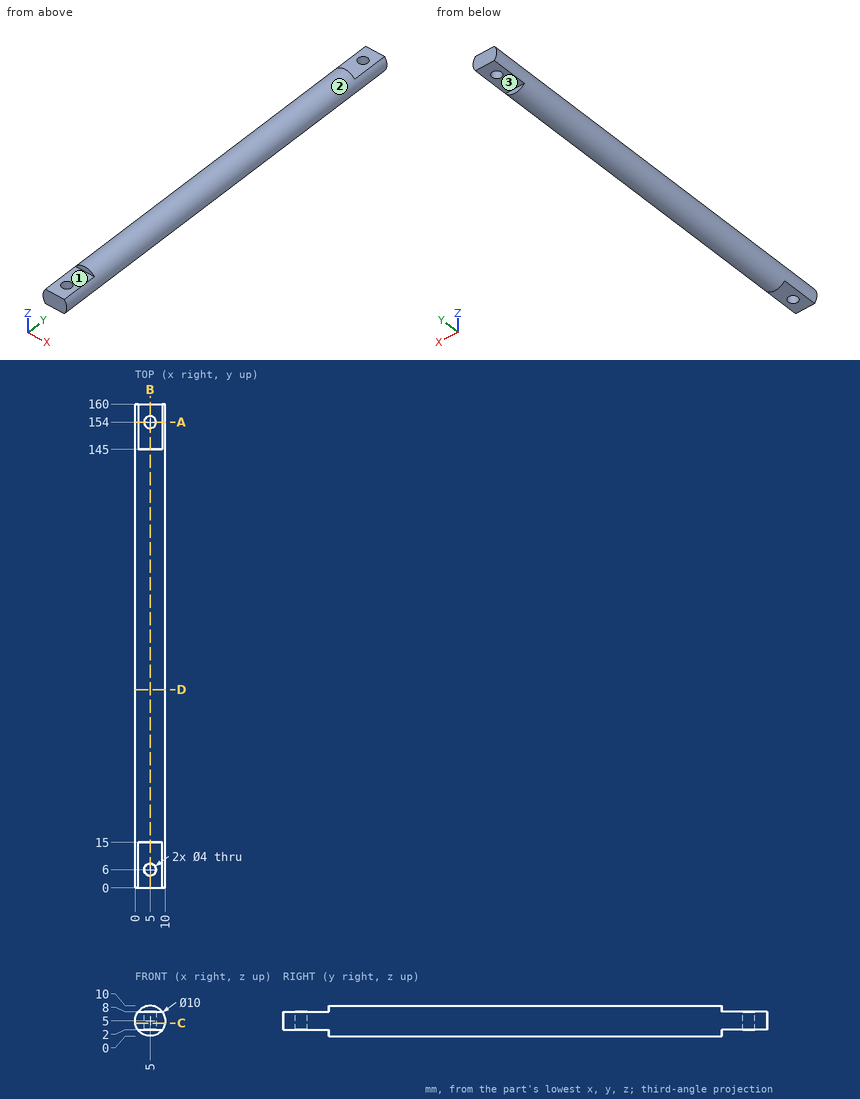
Answer from the drawing. Dimensions are ordinates in mm from the lowest x, y and z of the part. A direction names the side the tool comes from. Round coordinates to 2 decimals unless told otherwise and drop trailing zeros. Write each loop counter-clockwise with the first axis right and the second up, starting at its lowest first coordinate (ties: lowest second). Pieces come first, ordered by that corner, then holes. Notation, with made-up numbers: (73, -6.75) -> (99, -6.75) arc R8 cw to (99, 7.25) -> close; hole circle Ø5 at (-29.75, 49.25). An arc over 180 degrees is marked (long way). Answer in a Markdown table with one row per item. Add a question column.
1) Find section C-C, the plane z = 4.25. Determine the outline of the cut face in (x, y), and give its area (3 significant figures).
2) Which of the six approach directions +Z, -Z, +X, -X, +Y, -Y give full straight-line access (tool end or side, diameter ignored) to the marked faces 1, 2 and 3?
3) Find section B-B, the plane x = 5. Determine the outline of the cut face in (y, z), and give its area (3 significant figures).
4) Find section D-D, the plane y = 65.5. Determine the outline of the cut face in (x, z).
5) Find section A-A, the plane y = 154. Determine the outline of the cut face in (x, z), and give its area (3 significant figures).
6) Given P1, Ø4.5, axis at x = 5, y = 6, coming from the -Z side; P2, Ø2.5, axis at x = 4.5, y = 9.5, coming from the +Z side; P3, Ø0.6, axis at x = 3, z = 9, coming from the +Y side, each flat-ended and moving along its own axis, determine where each tip first touches the part or whether it passes through.
7) Consider line 1 (Y direction, x = 5, z = 5.4); line 2 (X direction, y = 6, z = 4.95); line 3 (Y direction, x = 4, z = 4.5). Determine where each line is inside the solid, lowest interval first.
Findings below:
| question | item | result |
|---|---|---|
| 1 | outline | (0.06, 0) -> (9.94, 0) -> (9.94, 160) -> (0.06, 160) -> close; hole circle Ø4 at (5, 6); hole circle Ø4 at (5, 154) |
| 1 | area | 1,560 mm² |
| 2 | face 1 | +Z, +X, -X, -Y |
| 2 | face 2 | +Y, -Y |
| 2 | face 3 | -Z, +X, -X, +Y |
| 3 | outline | (0, 2) -> (4, 2) -> (4, 8) -> (0, 8) -> close; (8, 2) -> (15, 2) -> (15, 0) -> (145, 0) -> (145, 2) -> (152, 2) -> (152, 8) -> (145, 8) -> (145, 10) -> (15, 10) -> (15, 8) -> (8, 8) -> close; (156, 2) -> (160, 2) -> (160, 8) -> (156, 8) -> close |
| 3 | area | 1,430 mm² |
| 4 | outline | circle Ø10 at (5, 5) |
| 5 | outline | (1, 2) -> (3, 2) -> (3, 8) -> (1, 8) arc R5 ccw to start; (7, 2) -> (9, 2) arc R5 ccw to (9, 8) -> (7, 8) -> close |
| 5 | area | 32.2 mm² |
| 6 | P1 | z = 2 |
| 6 | P2 | z = 8 |
| 6 | P3 | y = 145 |
| 7 | line 1 | 0 to 4, 8 to 152, 156 to 160 |
| 7 | line 2 | 0 to 3, 7 to 10 |
| 7 | line 3 | 0 to 4.27, 7.73 to 152.27, 155.73 to 160 |
